```python
from build123d import *

# Parameters (mm, degrees)
ESQUISSE1_R                  = 140
ESQUISSE1_R_2                = 97
BOSS_EXTRU_1_DEPTH           = 225
BOSS_EXTRU_2_START           = -32
ESQUISSE2_R                  = 23.5
BOSS_EXTRU_2_DEPTH           = 32
R_P_TITION_CIRCULAIRE1_COUNT = 3
SYM_TRIE3_START              = -32
SYM_TRIE3_COPY_1_SKETCH_R    = 23.5
SYM_TRIE3_COPY_1_DEPTH       = 32
SYM_TRIE3_COPY_2_SKETCH_R    = 23.5
SYM_TRIE3_COPY_2_DEPTH       = 32
ESQUISSE3_R                  = 100
BOSS_EXTRU_3_DEPTH           = 32
ESQUISSE4_R                  = 40
ENL_V_MAT_EXTRU_1_DEPTH      = 25
ESQUISSE5_R                  = 25
ENL_V_MAT_EXTRU_4_DEPTH      = 468.228990121
ESQUISSE6_R                  = 12.5
ENL_V_MAT_EXTRU_5_DEPTH      = 45
R_P_TITION_CIRCULAIRE2_COUNT = 6


with BuildPart() as part:
    # Esquisse1 → Boss.-Extru.1 (new body)
    with BuildSketch(Plane(origin=(0, 0, 0), x_dir=(0, 1, 0), z_dir=(0, 0, 1))):
        with Locations(Location((0, 0, 0), (0, 0, 270))):
            Circle(ESQUISSE1_R)
        with Locations(Location((0, 0, 0), (0, 0, 270))):
            Circle(ESQUISSE1_R_2, mode=Mode.SUBTRACT)
    extrude(amount=BOSS_EXTRU_1_DEPTH)

    # Esquisse2 → Boss.-Extru.2 (add)
    with BuildSketch(Plane.XY.offset(225).offset(BOSS_EXTRU_2_START)):
        with BuildLine():
            Line((-42.848913936, 175), (-42.848913936, 133.281546264))
            ThreePointArc((-42.848913936, 133.281546264), (7.657681027, 139.790414268), (57.151086064, 127.803573352))
            Line((57.151086064, 127.803573352), (57.151086064, 175))
            ThreePointArc((57.151086064, 175), (7.151086064, 225), (-42.848913936, 175))
        make_face()
        with Locations((7.151086064, 175)):
            Circle(ESQUISSE2_R, mode=Mode.SUBTRACT)
    boss_extru_2 = extrude(amount=BOSS_EXTRU_2_DEPTH)

    # Répétition circulaire1: Boss.-Extru.2 ×3 about axis
    r_p_tition_circulaire1_axis = Axis((0, 0, 0), (0, 0, 1))
    for i in range(1, R_P_TITION_CIRCULAIRE1_COUNT):
        add(boss_extru_2.rotate(r_p_tition_circulaire1_axis, i * 360 / R_P_TITION_CIRCULAIRE1_COUNT))

    # Symétrie3: Boss.-Extru.2 across plane
    add(boss_extru_2.mirror(Plane.XY.offset(112.5)))

    # Symétrie3 copy 1 sketch → Symétrie3 copy 1 (add)
    with BuildSketch(Plane(origin=(0, 0, 0), x_dir=(-0.4999999999999998, 0.8660254037844387, 0), z_dir=(0, 0, -1)).offset(SYM_TRIE3_START)):
        with BuildLine():
            Line((-42.848913936, -175), (-42.848913936, -133.281546264))
            ThreePointArc((-42.848913936, -133.281546264), (7.657681027, -139.790414268), (57.151086064, -127.803573352))
            Line((57.151086064, -127.803573352), (57.151086064, -175))
            ThreePointArc((57.151086064, -175), (7.151086064, -225), (-42.848913936, -175))
        make_face()
        with Locations((7.151086064, -175)):
            Circle(SYM_TRIE3_COPY_1_SKETCH_R, mode=Mode.SUBTRACT)
    extrude(amount=SYM_TRIE3_COPY_1_DEPTH)

    # Symétrie3 copy 2 sketch → Symétrie3 copy 2 (add)
    with BuildSketch(Plane(origin=(0, 0, 0), x_dir=(-0.5000000000000004, -0.8660254037844384, 0), z_dir=(0, 0, -1)).offset(SYM_TRIE3_START)):
        with BuildLine():
            Line((-42.848913936, -175), (-42.848913936, -133.281546264))
            ThreePointArc((-42.848913936, -133.281546264), (7.657681027, -139.790414268), (57.151086064, -127.803573352))
            Line((57.151086064, -127.803573352), (57.151086064, -175))
            ThreePointArc((57.151086064, -175), (7.151086064, -225), (-42.848913936, -175))
        make_face()
        with Locations((7.151086064, -175)):
            Circle(SYM_TRIE3_COPY_2_SKETCH_R, mode=Mode.SUBTRACT)
    extrude(amount=SYM_TRIE3_COPY_2_DEPTH)

    # Esquisse3 → Boss.-Extru.3 (add)
    with BuildSketch(Plane.YZ.offset(162)):
        with Locations(Location((37.953751354, 112.5, 0), (0, 0, 270))):
            Circle(ESQUISSE3_R)
    extrude(amount=-BOSS_EXTRU_3_DEPTH)

    # Esquisse4 → Enlèv. mat.-Extru.1 (cut)
    with BuildSketch(Plane.YZ.offset(162)):
        with Locations(Location((37.953751354, 112.5, 0), (0, 0, 270))):
            Circle(ESQUISSE4_R)
    extrude(amount=-ENL_V_MAT_EXTRU_1_DEPTH, mode=Mode.SUBTRACT)

    # Esquisse5 → Enlèv. mat.-Extru.4 (cut, through all)
    with BuildSketch(Plane.YZ.offset(137)):
        with Locations(Location((37.953751354, 112.5, 0), (0, 0, 270))):
            Circle(ESQUISSE5_R)
    extrude(amount=-ENL_V_MAT_EXTRU_4_DEPTH, mode=Mode.SUBTRACT)

    # Esquisse6 → Enlèv. mat.-Extru.5 (cut)
    with BuildSketch(Plane.YZ.offset(162)):
        with Locations(Location((37.503795096, 183.818066879, 0), (0, 0, 270))):
            Circle(ESQUISSE6_R)
    enl_v_mat_extru_5 = extrude(amount=-ENL_V_MAT_EXTRU_5_DEPTH, mode=Mode.SUBTRACT)

    # Répétition circulaire2: Enlèv. mat.-Extru.5 ×6 about axis
    r_p_tition_circulaire2_axis = Axis((0, 37.953751354, 112.5), (1, 0, 0))
    for i in range(1, R_P_TITION_CIRCULAIRE2_COUNT):
        add(enl_v_mat_extru_5.rotate(r_p_tition_circulaire2_axis, i * 360 / R_P_TITION_CIRCULAIRE2_COUNT), mode=Mode.SUBTRACT)


solid = part.part
```
Work out the finished part from the listing and answer in its coordinate system (mm). A direction names the side the tool comes from. Coordinates: 2 decimals unless noted, no trailing zeros. Loops run counter-clockwise (first coordinate to the right, second up) from the corner with the lowest first, then second, coordinate; pieces in that order, holes last. Notation, with made-up numbers: (61, -38) -> (65, -38) arc R17 cw to (65, -24) -> close; hole circle Ø1 at (87, 53). An arc over 180 degrees is marked (long way). Answer as CSV lines item,"result".
Q1. The part is cut by section D-D on x = 103.5. Write down the section's boundary in (y, z).
Findings:
outline,"(-125.75, 0) -> (94.27, 0) -> (94.27, 225) -> (-125.75, 225) -> (-125.75, 193) -> (-94.27, 193) -> (-94.27, 32) -> (-125.75, 32) -> close; hole circle Ø50 at (37.95, 112.5)"
Q2. The part is cut by section C-C on y = 120.5. Write down the section's boundary in (x, z).
Findings:
outline,"(-71.27, 0) -> (71.27, 0) -> (71.27, 225) -> (-71.27, 225) -> close; (130, 56.05) -> (162, 56.05) -> (162, 168.95) -> (130, 168.95) -> close"
Q3. For a pull along X with two mould halves and no side action, classify faces 1 (the face through (8.251, 224.988, 208.776)), 2 (the face through (-112.318, -114.325, 208.776)), 3 (the face through (-180, -82, 32)) as +X half, -X half, draft (parallel to the pull), parting line (faces both ways), or undercut.
Findings:
face 1,"parting line"
face 2,"undercut"
face 3,"draft"
Q4. A tool of negligible diameter and unlimited length cuts with its end or side. For faces 4 (the face through (161, -115, 32)), 5 (the face through (155.17, -40.11, 16.22)), 6 (the face through (57.151, 151, 16)), 7 (the face through (117, 38, 41)), from which of +Z, -Z, +X, -X, +Y, -Y can it reach the whole face along a straight path? Write none if from no direction.
Findings:
face 4,"+X, -Y"
face 5,"-Z, +X"
face 6,"+Z, -Z, +X, +Y"
face 7,"+X"
Q5. Each of these flat-tipped pins is pushed along its axis until it touches: pin 1 (20 mm diameter, centred on y = 41.5, z = 44, fed in from +X); pin 2 (12 mm diameter, centred on x = 135, z = 130.5, fed in from -Y); pin 3 (9.5 mm diameter, centred on y = 154, z = 204, fed in from +X). Where does it stop, or does it pass through?
Findings:
pin 1,"stops at x = 162"
pin 2,"stops at y = -61.32"
pin 3,"stops at x = 57.15"
Q6. The part is cut by section A-A on x = 0. Write down the section's boundary in (y, z), and give its area (3 significant figures).
Findings:
outline,"(-140, 0) -> (-97, 0) -> (-97, 225) -> (-140, 225) -> close; (97, 0) -> (152.61, 0) -> (152.61, 32) -> (140, 32) -> (140, 193) -> (152.61, 193) -> (152.61, 225) -> (97, 225) -> close; (197.39, 0) -> (224.49, 0) -> (224.49, 32) -> (197.39, 32) -> close; (197.39, 193) -> (224.49, 193) -> (224.49, 225) -> (197.39, 225) -> close"
area,"21,900 mm²"
Q7. Find the intervals of material crossed by probe 1 along Z at (x, y) = (152, -43); probe 2 along Y at (x, z) = (20.5, 197.5); probe 3 along X at (y, z) = (-56.5, 144.5), in increasing order.
Findings:
probe 1,"z = 0 to 32, 53.79 to 171.21, 193 to 225"
probe 2,"y = -138.49 to -94.81, 94.81 to 155.66, 194.34 to 223.19"
probe 3,"x = -128.09 to -78.85, 78.85 to 128.09, 130 to 162"
Q8. The part is cut by section B-B on z = 112.5. Write down the section's boundary in (x, y), and give its area (3 significant figures).
Findings:
outline,"(-139.4, 12.95) arc R140 ccw to (130, -51.96) -> (130, -62.05) -> (162, -62.05) -> (162, -2.05) -> (137, -2.05) -> (137, 12.95) -> (96.13, 12.95) arc R97 cw (long way) to (-96.13, 12.95) -> close; (-125.05, 62.95) -> (-73.8, 62.95) arc R97 cw to (73.8, 62.95) -> (125.05, 62.95) arc R140 ccw to start; (130, 62.95) -> (137, 62.95) -> (137, 77.95) -> (162, 77.95) -> (162, 137.95) -> (130, 137.95) -> close"
area,"31,000 mm²"
